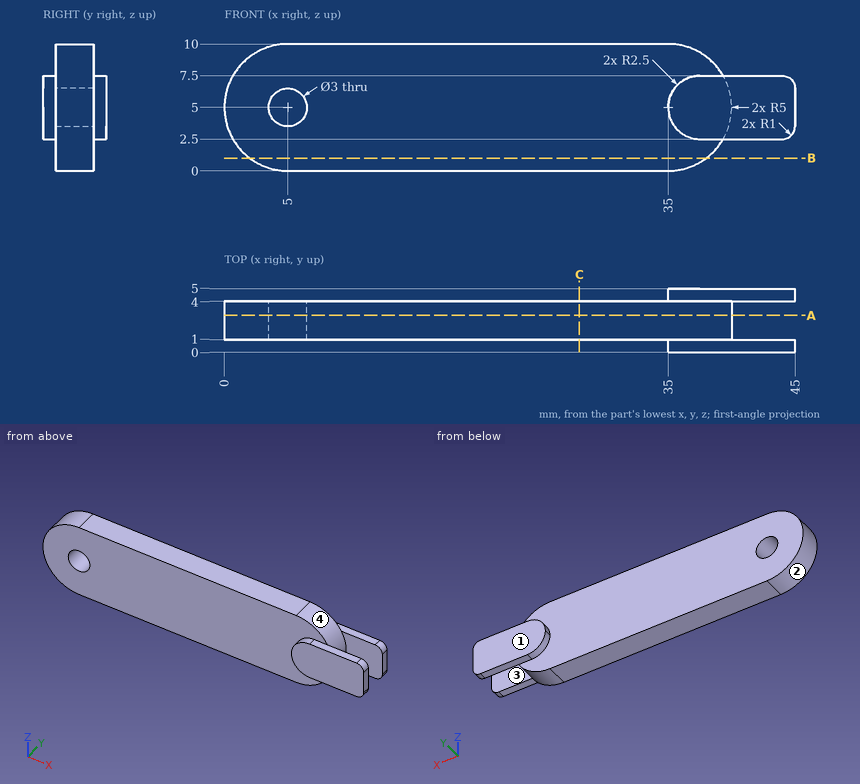
Input: dimensioned drawing with shaded views. Units: mm. Origin: part minimum x, y, z. Round coordinates to 2 decimals unless told otherwise and drop trailing zeros. Order: outer loops, then holes, each group sorted by start corner. A loop starts at its lowest first (then second) coordinate and runs counter-clockwise, first axis right, second up.
1. Cut plane C-C, the plane x = 28. Output: boundary loops of the cut face in (y, z).
The answers:
outline: (1, 0) - (4, 0) - (4, 10) - (1, 10) - close
2. Material intervals for line 1 (X direction, y = 2.75, z = 5); line 2 (Y direction, x = 14.5, z = 5); line 3 (X direction, y = 2.6, z = 6.25), sorted ascending.
The answers:
line 1: x = 0 to 3.5, 6.5 to 40
line 2: y = 1 to 4
line 3: x = 0.16 to 4.17, 5.83 to 39.84
3. Cut plane A-A, the plane y = 2.9. Output: boundary loops of the cut face in (x, z), then the cut area to 3 significant figures.
The answers:
outline: (5, 0) - (35, 0) arc R5 ccw to (35, 10) - (5, 10) arc R5 ccw to start; hole circle Ø3 at (5, 5)
area: 371 mm2
4. Cut plane B-B, the plane z = 1. Output: boundary loops of the cut face in (x, y).
The answers:
outline: (2, 1) - (38, 1) - (38, 4) - (2, 4) - close
5. Mould query, pull axis Y, two halves, no side actions, for the marked faces 1, 2, 3 and 4. Classes: released by +Y, released by -Y, zero draft, split by the parting line, or undercut.
The answers:
face 1: released by +Y
face 2: zero draft
face 3: undercut
face 4: undercut
6. Pin query (flat end, axial travel): P1, Ø2.5, axis at x = 43, z = 4, coming from the -Y side; P2, Ø6, axis at x = 7, z = 1.5, coming from the +Y side; P3, Ø2, axis at y = 4.5, z = 7.5, coming from the -X side; P4, Ø1, axis at x = 15, z = 8.5, coming from the -Y side. Return the tip coordinate at first contact, or that it passes through.
The answers:
P1: stops at y = 0
P2: stops at y = 4
P3: stops at x = 0.27
P4: stops at y = 1
